Verification items for the finished model (mm, model axes). A direction names the side the tool comes from. Give positions to 0.01 mm unless a question says otherwise; leave off trailing zeros. Loops run counter-clockwise (first coordinate to the right, second up) from the corner with the lowest first, then second, coordinate; pieces in that order, holes last. Notation, with made-up numbers: (11.25, 39.25) -> (30.25, 39.25) arc R26 ccw to (30.25, 53.25) -> close; hole circle Ø8 at (47.25, -37). An arc over 180 degrees is marked (long way). Answer in a Markdown table with one row per item. Add a question column.
Q1. Section check B-B on z = 1.05. Give the number of separate pieces and of enclosed holes in the cut face, and give its area (3 significant figures).
Q2. Section check D-D on x = 82.5. Enter the section's corners in (y, z), and give its area (3 significant figures).
Q3. Gauge pin test, flat ends, axial feed: P1, Ø12, axis at x = 0, y = 0, coming from the +Z side; P2, Ø1.5, axis at y = 62, z = 1.5, coming from the -X side; P3, Ø1.5, axis at y = 30, z = 2, coming from the +X side. Record the tip position at first contact, or that the pin passes through.
Q4. Release check for a two-part mould opening along X. For faces 3 (the face through (-17.105, -10.383, 1.479)), 4 (the face through (21, 1, 3)), 5 (the face through (-13.26, 100.992, 1.479)) record: pulls with the +X half, pulls with the -X half, needs draft (parallel to the pull), parting line crosses it, or undercut.
Q5. Section check C-C on x = -84. Enter the section's corners in (y, z).
Q6. Section check A-A on y = 24. Enter the section's corners in (x, z), and give its area (3 significant figures).
Q7. Set-up check for faces 1 (the face through (21, 1, 0)), 2 (the face through (64.824, -37.634, 1.479)): record each of +Z, -Z, +X, -X, +Y, -Y from which the full face is reachable in a straight line by a thin tool's end or side.
Q8. Material ranges on probe 1 along Y at (x, z) = (0, 1.95); probe 2 along X at (y, z) = (-4.5, 1.65); probe 3 along X at (y, z) = (-38, 2.05), recorded low to high.
```python
from build123d import *

# Parameters (mm, degrees)
SKETCH1_R           = 101.859163579
SKETCH1_R_2         = 2
SKETCH1_R_3         = 10
BOSS_EXTRUDE1_DEPTH = 3


with BuildPart() as part:
    # Sketch1 → Boss-Extrude1 (new body)
    with BuildSketch(Plane.XY):
        Circle(SKETCH1_R)
        with Locations((0, 90)):
            Circle(SKETCH1_R_2, mode=Mode.SUBTRACT)
        with Locations((77.942286341, 45)):
            Circle(SKETCH1_R_2, mode=Mode.SUBTRACT)
        with Locations((77.942286341, -45)):
            Circle(SKETCH1_R_2, mode=Mode.SUBTRACT)
        with Locations((0, -90)):
            Circle(SKETCH1_R_2, mode=Mode.SUBTRACT)
        with Locations((-77.942286341, -45)):
            Circle(SKETCH1_R_2, mode=Mode.SUBTRACT)
        with Locations((-77.942286341, 45)):
            Circle(SKETCH1_R_2, mode=Mode.SUBTRACT)
        Circle(SKETCH1_R_3, mode=Mode.SUBTRACT)
        with BuildLine():
            Line((-20, 74.95508592), (-20, 40))
            ThreePointArc((-20, 40), (0, 20), (20, 40))
            Line((20, 40), (20, 74.95508592))
            ThreePointArc((20, 74.95508592), (17.236067977, 79.427221875), (12, 78.95508592))
            ThreePointArc((12, 78.95508592), (0, 74.95508592), (-12, 78.95508592))
            ThreePointArc((-12, 78.95508592), (-17.236067977, 79.427221875), (-20, 74.95508592))
        make_face(mode=Mode.SUBTRACT)
        with BuildLine():
            Line((74.91300855, -20.157034884), (44.641016151, -2.679491924))
            ThreePointArc((44.641016151, -2.679491924), (17.320508076, -10), (24.641016151, -37.320508076))
            Line((24.641016151, -37.320508076), (54.91300855, -54.798051036))
            ThreePointArc((54.91300855, -54.798051036), (60.167957907, -54.640483667), (62.377110165, -49.869847805))
            ThreePointArc((62.377110165, -49.869847805), (64.91300855, -37.47754296), (74.377110165, -29.085238115))
            ThreePointArc((74.377110165, -29.085238115), (77.404025885, -24.786738208), (74.91300855, -20.157034884))
        make_face(mode=Mode.SUBTRACT)
        with BuildLine():
            Line((-54.91300855, -54.798051036), (-24.641016151, -37.320508076))
            ThreePointArc((-24.641016151, -37.320508076), (-17.320508076, -10), (-44.641016151, -2.679491924))
            Line((-44.641016151, -2.679491924), (-74.91300855, -20.157034884))
            ThreePointArc((-74.91300855, -20.157034884), (-77.404025885, -24.786738208), (-74.377110165, -29.085238115))
            ThreePointArc((-74.377110165, -29.085238115), (-64.91300855, -37.47754296), (-62.377110165, -49.869847805))
            ThreePointArc((-62.377110165, -49.869847805), (-60.167957907, -54.640483667), (-54.91300855, -54.798051036))
        make_face(mode=Mode.SUBTRACT)
    extrude(amount=BOSS_EXTRUDE1_DEPTH)


solid = part.part
```
Taken from the geometry:
| question | item | result |
|---|---|---|
| 1 | separate pieces | 1 |
| 1 | enclosed holes | 10 |
| 1 | area | 25,800 mm² |
| 2 | outline | (-59.74, 0) -> (59.74, 0) -> (59.74, 3) -> (-59.74, 3) -> close |
| 2 | area | 358 mm² |
| 3 | P1 | passes through |
| 3 | P2 | stops at x = -81.39 |
| 3 | P3 | stops at x = 97.57 |
| 4 | face 3 | undercut |
| 4 | face 4 | needs draft |
| 4 | face 5 | parting line crosses it |
| 5 | outline | (-57.61, 0) -> (57.61, 0) -> (57.61, 3) -> (-57.61, 3) -> close |
| 6 | outline | (-98.99, 0) -> (-12, 0) -> (-12, 3) -> (-98.99, 3) -> close; (12, 0) -> (98.99, 0) -> (98.99, 3) -> (12, 3) -> close |
| 6 | area | 522 mm² |
| 7 | face 1 | -Z, +X, -X, +Y, -Y |
| 7 | face 2 | +Z, -Z |
| 8 | probe 1 | y = -101.86 to -92, -88 to -10, 10 to 20, 74.96 to 88, 92 to 101.86 |
| 8 | probe 2 | x = -101.76 to -47.79, -22 to -8.93, 8.93 to 22, 47.79 to 101.76 |
| 8 | probe 3 | x = -94.51 to -64.62, -25.82 to 25.82, 64.62 to 94.51 |
